Geometry: final body of the model. Coordinates: model frame, mm. Face numbers are marked on the shaded views. A direction names the side the tool comes from. Round coordinates to 2 decimals unless told otherwise and drop trailing zeros. Write each loop counter-clockwise with the first axis right and the second up, starting at its lowest first coordinate (ties: lowest second). Pieces come first, ordered by that corner, then holes. Notation, with made-up numbers: M -38.75,21 L -15.75,21 A18 ccw -15.75,40 Z; hole C 84.25,-20.75 d7. An arc over 180 degrees is marked long. Use one line per item in the form item = value. Start each with the question number.
Item 1: Ray query, probe 1 along Y at (x, z) = (0, 3); probe 2 along Y at (x, z) = (0, 13.25); probe 3 along X at (y, z) = (-2, 8.75). Return the intervals inside material, ascending.
Item 2: Section query A-A (y = 0). Return loops of the section in (x, z), and give its area (3 significant figures).
Item 3: Section query D-D (y = -24). Return loops of the section in (x, z).
Item 4: Pull-direction query (Y, two-part tool) for the marked faces 1, 2 and 3; classes: pulls with the +Y half, pulls with the -Y half, needs draft (parallel to the pull), parting line crosses it, or undercut.
Item 5: Section query C-C (z = 13.75). Return loops of the section in (x, y).
Item 6: Reachability of the marked faces 4 and 5 from +Z, -Z, +X, -X, +Y, -Y: full face, straight path, thin tool, end or side. Return the list, or none.
Item 7: Pin query (flat end, axial travel): pin 1 Ø9 at (x, y) = (0, 25.15) entering from -Z; pin 2 Ø8 at (x, z) = (4, 4) entering from -Y; pin 3 Ø5 at (y, z) = (13, 7.5) entering from +X. Return the tip coordinate at first contact, or that it passes through.
Item 8: Section query B-B (x = -25.15). Return loops of the section in (y, z).
from build123d import *

# Parameters (mm, degrees)
SKETCH1_R           = 30
BOSS_EXTRUDE1_DEPTH = 15
SKETCH2_R           = 2.2
CUT_EXTRUDE1_DEPTH  = 15
SKETCH3_R           = 4
CUT_EXTRUDE2_DEPTH  = 4.5
SKETCH5_R           = 8
BOSS_EXTRUDE2_DEPTH = 1.5
SKETCH8_R           = 3.25
CUT_EXTRUDE3_DEPTH  = 7


with BuildPart() as part:
    # Sketch1 → Boss-Extrude1 (new body)
    with BuildSketch(Plane.XY):
        Circle(SKETCH1_R)
    extrude(amount=BOSS_EXTRUDE1_DEPTH)

    # Sketch2 → Cut-Extrude1 (cut)
    with BuildSketch(Plane.XY):
        with Locations((0, 25.15)):
            Circle(SKETCH2_R)
        with Locations((25.15, 0)):
            Circle(SKETCH2_R)
        with Locations((0, -25.15)):
            Circle(SKETCH2_R)
        with Locations((-25.15, 0)):
            Circle(SKETCH2_R)
    extrude(amount=CUT_EXTRUDE1_DEPTH, mode=Mode.SUBTRACT)

    # Sketch3 → Cut-Extrude2 (cut)
    with BuildSketch(Plane.XY):
        with Locations((0, 25.15)):
            Circle(SKETCH3_R)
        with Locations((25.15, 0)):
            Circle(SKETCH3_R)
        with Locations((0, -25.15)):
            Circle(SKETCH3_R)
        with Locations((-25.15, 0)):
            Circle(SKETCH3_R)
    extrude(amount=CUT_EXTRUDE2_DEPTH, mode=Mode.SUBTRACT)

    # Sketch5 → Boss-Extrude2 (add)
    with BuildSketch(Plane.XY):
        Circle(SKETCH5_R)
    extrude(amount=-BOSS_EXTRUDE2_DEPTH)

    # Sketch8 → Cut-Extrude3 (cut)
    with BuildSketch(Plane.XY.offset(-1.5)):
        Circle(SKETCH8_R)
    extrude(amount=CUT_EXTRUDE3_DEPTH, mode=Mode.SUBTRACT)


solid = part.part
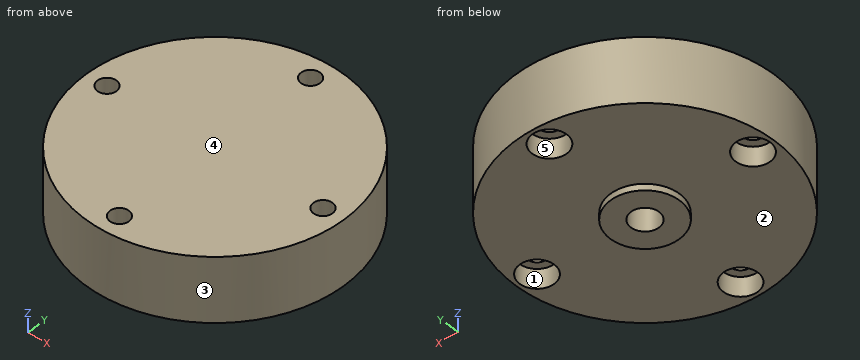
Working result:
q1.probe_1 = -30 to -29.15, -21.15 to -3.25, 3.25 to 21.15, 29.15 to 30
q1.probe_2 = -30 to -27.35, -22.95 to 22.95, 27.35 to 30
q1.probe_3 = -29.93 to -26.07, -24.23 to 24.23, 26.07 to 29.93
q2.outline = M -30,0 L -29.15,0 L -29.15,4.5 L -27.35,4.5 L -27.35,15 L -30,15 Z; M -22.95,4.5 L -21.15,4.5 L -21.15,0 L -8,0 L -8,-1.5 L -3.25,-1.5 L -3.25,5.5 L 3.25,5.5 L 3.25,-1.5 L 8,-1.5 L 8,0 L 21.15,0 L 21.15,4.5 L 22.95,4.5 L 22.95,15 L -22.95,15 Z; M 27.35,4.5 L 29.15,4.5 L 29.15,0 L 30,0 L 30,15 L 27.35,15 Z
q2.area = 714 mm²
q3.outline = M -18,0 L -3.83,0 L -3.83,4.5 L -1.88,4.5 L -1.88,15 L -18,15 Z; M 1.88,4.5 L 3.83,4.5 L 3.83,0 L 18,0 L 18,15 L 1.88,15 Z
q4.face_1 = undercut
q4.face_2 = needs draft
q4.face_3 = parting line crosses it
q5.outline = C 0,0 d60; hole C -25.15,0 d4.4; hole C 0,-25.15 d4.4; hole C 0,25.15 d4.4; hole C 25.15,0 d4.4
q6.face_4 = +Z, +X, -X, +Y, -Y
q6.face_5 = -Z
q7.pin_1 = 0
q7.pin_2 = -30
q7.pin_3 = 28.1
q8.outline = M -16.35,0 L -4,0 L -4,4.5 L -2.2,4.5 L -2.2,15 L -16.35,15 Z; M 2.2,4.5 L 4,4.5 L 4,0 L 16.35,0 L 16.35,15 L 2.2,15 Z
